Read the model definition and answer for the solid it produces. Units are mm, in the model's axes. A direction names the side the tool comes from. Round coordinates to 2 decimals unless told otherwise and drop trailing zeros. Write each loop counter-clockwise with the first axis right and the second up, starting at its lowest first coordinate (ties: lowest second). Pieces come first, ordered by that corner, then holes. Notation, with made-up numbers: (13.25, 36) - (52.25, 36) arc R32 ccw to (52.25, 71) - close; hole circle Ø9 at (-12, -20). An arc over 180 degrees is marked (long way). One line per item, written item: value. Start each with the question number.
(1) Find the intervals of material crossed by L1, parallel to Z at x = 9, y = 40.5 (3 decimals); L2, parallel to Y at x = 28, z = 26; L3, parallel to Z at x = 57.5, y = 23, in increasing order.
(2) A cutting plane is placed at B-B, the plane y = -52. Determine the outline of the cut face in (x, z) (3 decimals).
(3) For faces 1 (the face through (32.39, -16.79, 51.63)), 2 (the face through (46, -25.4, 42)), 3 (the face through (45.8, -0.4, 38.1)), 4 (the face through (46, 25.4, 42)), determine the directions among +Z, -Z, +X, -X, +Y, -Y from which every point of the face is accessible in a straight line to the end or side of a thin tool.
(4) A cutting plane is placed at A-A, the plane x = 65.5. Determine the outline of the cut face in (y, z) (3 decimals).
(5) Flat-ended cylindrical pins translate along their axes: pin 1 Ø1 at (x, y) = (29.5, -21.5) entering from +Z; pin 2 Ø5 at (x, y) = (94, 12) entering from -Z; pin 3 Ø1 at (x, y) = (9, 48.5) entering from +Z (3 decimals). Find the tip coordinate at first contact, or state that the pin passes through.
from build123d import *

# Parameters (mm, degrees)
F1_DEPTH = 63.5
F0_W     = 25.4
F0_H     = 19.05
F2_DEPTH = 25.4
F3_DEPTH = 7.9375
F5_R     = 6.35


with BuildPart() as f1:
    # F0 (on Front) → F1 (new body, symmetric)
    with BuildSketch(Plane.XZ):
        Polygon((-41.275, 9.525), (-41.275, -9.525), (41.275, -9.525), (41.275, 9.525), (22.225, 9.525), align=None)
    extrude(amount=F1_DEPTH, both=True)

    # F0 (on Front) → F2 (join, symmetric)
    with BuildSketch(Plane.XZ):
        with BuildLine():
            Line((22.225, 9.525), (41.275, 9.525))
            Line((41.275, 9.525), (41.275, 27.0002))
            ThreePointArc((41.275, 27.0002), (45.9246798487, 38.2255201513), (57.15, 42.8752))
            Line((57.15, 42.8752), (60.325, 42.8752))
            Line((60.325, 42.8752), (60.325, 61.9252))
            Line((60.325, 61.9252), (57.15, 61.9252))
            add(Edge.make_bspline(
                [(56.2167130803, 61.912727845), (56.5273358461, 61.9178208633), (56.8384328672, 61.9219806407), (57.15, 61.9252)],
                knots=[110.8966420493, 110.8966420493, 110.8966420493, 110.8966420493, 111.5045361635, 111.5045361635, 111.5045361635, 111.5045361635], degree=3))
            ThreePointArc((56.2167130803, 61.912727845), (32.1265043342, 51.3637032306), (22.225, 27.0002))
            Line((22.225, 27.0002), (22.225, 9.525))
        make_face()
        with Locations((73.025, 52.4002)):
            Rectangle(F0_W, F0_H)
    extrude(amount=F2_DEPTH, both=True)

    # F0 (on Front) → F3 (join, symmetric)
    with BuildSketch(Plane.XZ):
        with BuildLine():
            add(Edge.make_bspline(
                [(-41.275, 9.525), (-41.332462601, 28.9964285063), (-0.4494412016, 60.9836209238), (56.2167130803, 61.912727845)],
                knots=[0, 0, 0, 0, 110.8966420493, 110.8966420493, 110.8966420493, 110.8966420493], degree=3))
            Line((-41.275, 9.525), (22.225, 9.525))
            Line((22.225, 9.525), (22.225, 27.0002))
            ThreePointArc((22.225, 27.0002), (32.1265043342, 51.3637032306), (56.2167130803, 61.912727845))
        make_face()
    extrude(amount=F3_DEPTH, both=True)

    # F0 (on Front) → F4 (revolve)
    with BuildSketch(Plane.XZ):
        Polygon((85.725, 66.675), (85.725, 61.9252), (85.725, 42.8752), (85.725, 38.1), (111.125, 38.1), (111.125, 66.675), align=None)
    revolve(axis=Axis((85.725, 0, 52.3875), (0, 0, 1)))

    # F5
    f5_edges = [f1.edges().sort_by_distance(p)[0] for p in [
        (41.275, -63.5, 0),
        (-41.275, -63.5, 0),
        (-41.275, 63.5, 0),
    ]]
    fillet(f5_edges, radius=F5_R)


solid = f1.part
Here are the results:
1. L1: -9.525 to 9.525
1. L2: -25.4 to 25.4
1. L3: 42.88 to 61.93
2. outline: (-41.275, -9.525) - (41.275, -9.525) - (41.275, 9.525) - (-41.275, 9.525) - close
3. face 1: +Z, -X, -Y
3. face 2: +Z, +X, -X, -Y
3. face 3: -Z, +Y, -Y
3. face 4: +Z, +X, -X, +Y
4. outline: (-25.4, 42.875) - (-15.366, 42.875) - (-15.366, 38.1) - (15.366, 38.1) - (15.366, 42.875) - (25.4, 42.875) - (25.4, 61.925) - (15.366, 61.925) - (15.366, 66.675) - (-15.366, 66.675) - (-15.366, 61.925) - (-25.4, 61.925) - close
5. pin 1: z = 48.97
5. pin 2: z = 38.1
5. pin 3: z = 9.525
